Can you work these out from the model? Positions are in its coordinate system, mm. A direction names the side the tool comes from. Give positions to 0.01 mm unless a question says otherwise; leave off trailing zeros. Order: outer loops, then holes, each group sorted by start corner. A loop starts at its lowest first (then second) coordinate and runs counter-clockwise, first axis right, second up. Notation, with made-up numbers: M 58,59.25 L 98,59.25 A23 cw 98,84.25 Z; hole C -3.5,78 d5. An arc over 180 degrees is marked long. Use one line per item in the form item = value. Start each with the question number.
1. I need wall thicknesses on L1, parallel to Y at x = 109, z = 1.3; L2, parallel to X at y = 79.5, z = 2.6; L3, parallel to X at y = 73.5, z = 0.85. Which ranges of each line are inside material? Lowest first, please.
2. Will these pins go through, and if not, where does the flat tip stop? P1, Ø3.5, axis at x = 109, y = 7.96, coming from the -Z side; P2, Ø2, axis at x = 80.5, z = 1, coming from the +Y side.
3. For faces 1 (the face through (73, 53.484, 2)), 2 (the face through (39, -26, 2)), which set-ups out of +Z, -Z, +X, -X, +Y, -Y let a thin tool reach every point of the face, with its end or its side?
4. I want a section at A-A, the plane y = 40. List the corners of the cut face in (x, z) for me.
5. I want a section at C-C, the plane y = 109. List the corners of the cut face in (x, z) for me.
6. We'd pull the mould along Y, two halves only. Please class faces 3 (the face through (106.14, 8.86, 1.97)), 4 (the face through (29, 123.484, 2)), 5 (the face through (141.001, 48, 2)): +Y half, -Y half, draft (parallel to the pull), parting line (faces both ways), or undercut.
7. I want a section at D-D, the plane z = 2. Count the separate pieces of the cut face and the enclosed holes in it, and give its area (3 significant figures).
8. I want a section at B-B, the plane x = 36. List the corners of the cut face in (y, z) for me, and give its area (3 significant figures).
```python
from build123d import *

# Parameters (mm, degrees)
SKETCH_1_R          = 2
EXTRUDE_1_DEPTH     = 4
SKETCH_2_R          = 2
CUT_EXTRUDE_1_DEPTH = 26
EXTRUDE_3_DEPTH     = 4
FILLET_1_R          = 4
FILLET_2_R          = 4
SKETCH_5_W          = 10
SKETCH_5_H          = 14
EXTRUDE_4_DEPTH     = 4
FILLET_3_R          = 4
FILLET_1_2_DEPTH    = 4
CUT_EXTRUDE_2_DEPTH = 10
SKETCH_7_R          = 3
CUT_EXTRUDE_3_DEPTH = 10
CUT_EXTRUDE_4_DEPTH = 10
SKETCH_9_W          = 20
SKETCH_9_H          = 70
SKETCH_9_R          = 3
CUT_EXTRUDE_5_DEPTH = 10
CUT_EXTRUDE_6_DEPTH = 10


with BuildPart() as part:
    # 草图1 → 凸台-拉伸1 (new body)
    with BuildSketch(Plane.XY):
        with BuildLine():
            Line((0, -30), (0, 87))
            Line((0, 87), (-8, 87))
            Line((-8, 87), (-8, 95))
            Line((-8, 95), (0, 95))
            Line((0, 95), (0, 155))
            Line((0, 155), (-20, 155))
            Line((-20, 155), (-20, 180))
            Line((-20, 180), (-8, 180))
            ThreePointArc((-8, 180), (-0.928932188, 182.928932188), (2, 190))
            Line((2, 190), (2, 212))
            Line((2, 212), (10, 212))
            Line((10, 212), (10, 190))
            ThreePointArc((10, 190), (12.928932188, 182.928932188), (20, 180))
            Line((20, 180), (72.5, 180))
            Line((72.5, 180), (125, 180))
            ThreePointArc((125, 180), (132.071067812, 182.928932188), (135, 190))
            Line((135, 190), (135, 212))
            Line((135, 212), (143, 212))
            Line((143, 212), (143, 190))
            ThreePointArc((143, 190), (145.928932188, 182.928932188), (153, 180))
            Line((153, 180), (165, 180))
            Line((165, 180), (165, 155))
            Line((165, 155), (145, 155))
            Line((145, 155), (145, 95))
            Line((145, 95), (153, 95))
            Line((153, 95), (153, 87))
            Line((153, 87), (145, 87))
            Line((145, 87), (145, -30))
            Line((145, -30), (0, -30))
        make_face()
        with Locations((139, 208)):
            Circle(SKETCH_1_R, mode=Mode.SUBTRACT)
        with Locations(Location((149, 91, 0), (0, 0, 180))):
            Circle(SKETCH_1_R, mode=Mode.SUBTRACT)
        with Locations(Location((9, 40, 0), (0, 0, 180))):
            Circle(SKETCH_1_R, mode=Mode.SUBTRACT)
        with Locations(Location((9, 120, 0), (0, 0, 180))):
            Circle(SKETCH_1_R, mode=Mode.SUBTRACT)
        with Locations((-4, 91)):
            Circle(SKETCH_1_R, mode=Mode.SUBTRACT)
        with Locations(Location((6, 208, 0), (0, 0, 180))):
            Circle(SKETCH_1_R, mode=Mode.SUBTRACT)
        with Locations((136, 120)):
            Circle(SKETCH_1_R, mode=Mode.SUBTRACT)
        with Locations((136, 40)):
            Circle(SKETCH_1_R, mode=Mode.SUBTRACT)
    extrude(amount=EXTRUDE_1_DEPTH)

    # 草图2 → 切除-拉伸1 (cut)
    with BuildSketch(Plane(origin=(0, 0, 0), x_dir=(-1, 0, 0), z_dir=(0, 0, -1))):
        with Locations((-90.5, 176)):
            Circle(SKETCH_2_R)
        with Locations((-82.5, 176)):
            Circle(SKETCH_2_R)
        with Locations((-62.5, 176)):
            Circle(SKETCH_2_R)
        with Locations((-54.5, 176)):
            Circle(SKETCH_2_R)
    extrude(amount=-CUT_EXTRUDE_1_DEPTH, mode=Mode.SUBTRACT)

    # 草图4 → 凸台-拉伸3 (add)
    with BuildSketch(Plane(origin=(0, 0, 0), x_dir=(-1, 0, 0), z_dir=(0, 0, -1))):
        with BuildLine():
            Line((-102.5, 194), (-102.5, 204.972470671))
            Line((-102.5, 204.972470671), (-99, 215.944941341))
            Line((-99, 215.944941341), (-95.5, 215.944941341))
            ThreePointArc((-95.5, 215.944941341), (-92.121980777, 211.957020041), (-89.03099134, 207.742721229))
            ThreePointArc((-89.03099134, 207.742721229), (-72.5, 199), (-55.96900866, 207.742721229))
            ThreePointArc((-55.96900866, 207.742721229), (-52.878019223, 211.957020041), (-49.5, 215.944941341))
            Line((-49.5, 215.944941341), (-46, 215.944941341))
            Line((-46, 215.944941341), (-42.5, 204.972470671))
            Line((-42.5, 204.972470671), (-42.5, 194))
            Line((-42.5, 194), (-42.5, 180))
            Line((-42.5, 180), (-49.5, 180))
            Line((-49.5, 180), (-49.5, 194))
            Line((-49.5, 194), (-95.5, 194))
            Line((-95.5, 194), (-95.5, 180))
            Line((-95.5, 180), (-102.5, 180))
            Line((-102.5, 180), (-102.5, 194))
        make_face()
    extrude(amount=-EXTRUDE_3_DEPTH)

    # Fillet 1
    fillet_1_edges = [part.edges().sort_by_distance(p)[0] for p in [
        (102.5, 180, 2),
    ]]
    fillet(fillet_1_edges, radius=FILLET_1_R)

    # 圆角2
    fillet_2_edges = [part.edges().sort_by_distance(p)[0] for p in [
        (42.5, 180, 2),
    ]]
    fillet(fillet_2_edges, radius=FILLET_2_R)

    # 草图5 → 凸台-拉伸4 (add)
    with BuildSketch(Plane(origin=(0, 0, 0), x_dir=(-1, 0, 0), z_dir=(0, 0, -1))):
        with Locations((-71.485667886, 187)):
            Rectangle(SKETCH_5_W, SKETCH_5_H)
    extrude(amount=-EXTRUDE_4_DEPTH)

    # 圆角3
    fillet_3_edges = [part.edges().sort_by_distance(p)[0] for p in [
        (0, 95, 2),
    ]]
    fillet(fillet_3_edges, radius=FILLET_3_R)

    # Fillet 1 2: read off the stored shape, not the designer's step
    # Fillet 1 2 outline → Fillet 1 2 (add)
    with BuildSketch(Plane.XY):
        with BuildLine():
            add(Edge.make_bspline(
                [(0, 85), (0, 87), (-2, 87)],
                knots=[0, 0, 0, 1, 1, 1], degree=2, weights=[1, 0.707106781, 1]))
            Line((0, 85), (0, 87))
            Line((0, 87), (-2, 87))
        make_face()
        with BuildLine():
            add(Edge.make_bspline(
                [(145, 97), (145, 95), (147, 95)],
                knots=[0, 0, 0, 1, 1, 1], degree=2, weights=[1, 0.707106781, 1]))
            Line((145, 97), (145, 95))
            Line((145, 95), (147, 95))
        make_face()
        with BuildLine():
            add(Edge.make_bspline(
                [(147, 87), (145, 87), (145, 85)],
                knots=[0, 0, 0, 1, 1, 1], degree=2, weights=[1, 0.707106781, 1]))
            Line((147, 87), (145, 87))
            Line((145, 87), (145, 85))
        make_face()
    extrude(amount=FILLET_1_2_DEPTH)

    # 草图6 → 切除-拉伸2 (cut)
    with BuildSketch(Plane(origin=(0, 0, 0), x_dir=(-1, 0, 0), z_dir=(0, 0, -1))):
        with BuildLine():
            Line((-145, 126), (0, 127))
            ThreePointArc((0, 127), (86.5779564, 788.380122484), (-240.522742442, 207.067348009))
            Line((-240.522742442, 207.067348009), (-145, 126))
        make_face()
        Polygon((-145, 97), (-145, 85), (-184.843069779, 78.009614434), (-187.688323439, 115.332647741), align=None)
        Polygon((0, 85), (0, 99), (22.414932697, 115.332647741), (70.043948421, 78.009614434), align=None)
    extrude(amount=-CUT_EXTRUDE_2_DEPTH, mode=Mode.SUBTRACT)

    # 草图7 → 切除-拉伸3 (cut)
    with BuildSketch(Plane(origin=(0, 0, 0), x_dir=(-1, 0, 0), z_dir=(0, 0, -1))):
        with Locations((-109, 7.960589548)):
            Circle(SKETCH_7_R)
        with Locations((-36, 7.960589548)):
            Circle(SKETCH_7_R)
        with Locations((-109, -26.039410452)):
            Circle(SKETCH_7_R)
        with Locations((-36, -26.039410452)):
            Circle(SKETCH_7_R)
        with Locations((-124.840103492, 79.073280951)):
            Circle(SKETCH_7_R)
        with Locations((-124.840103492, 21.073280951)):
            Circle(SKETCH_7_R)
        with Locations((-95.840103492, 21.073280951)):
            Circle(SKETCH_7_R)
        with Locations((-95.840103492, 79.073280951)):
            Circle(SKETCH_7_R)
        with Locations((-65.68273437, 95.743302343)):
            Circle(SKETCH_7_R)
        with Locations((-65.68273437, 12.743302343)):
            Circle(SKETCH_7_R)
        with Locations((-17.742400545, 17.739740347)):
            Circle(SKETCH_7_R)
        with Locations((-17.742400545, 92.739740347)):
            Circle(SKETCH_7_R)
    extrude(amount=-CUT_EXTRUDE_3_DEPTH, mode=Mode.SUBTRACT)

    # 草图8 → 切除-拉伸4 (cut)
    with BuildSketch(Plane(origin=(0, 0, 0), x_dir=(-1, 0, 0), z_dir=(0, 0, -1))):
        Polygon((-154.568758674, 123.48356313), (9.260166048, 123.48356313), (22.383573851, 133.739706362), (-120.787265427, 138.710916059), align=None)
    extrude(amount=-CUT_EXTRUDE_4_DEPTH, mode=Mode.SUBTRACT)

    # 草图9 → 切除-拉伸5 (cut)
    # profile 1 of 2: a face of its own
    with BuildSketch(Plane(origin=(0, 0, 0), x_dir=(-1, 0, 0), z_dir=(0, 0, -1))):
        with Locations((-82.5, 88.48356313)):
            Rectangle(SKETCH_9_W, SKETCH_9_H)
    # profile 2 of 2: a face of its own
    with BuildSketch(Plane(origin=(0, 0, 0), x_dir=(-1, 0, 0), z_dir=(0, 0, -1))):
        with Locations((-62.5, 88.48356313)):
            Rectangle(SKETCH_9_W, SKETCH_9_H)
        with Locations((-65.68273437, 95.743302343)):
            Circle(SKETCH_9_R, mode=Mode.SUBTRACT)
    extrude(amount=-CUT_EXTRUDE_5_DEPTH, mode=Mode.SUBTRACT)

    # 草图10 → 切除-拉伸6 (cut)
    with BuildSketch(Plane(origin=(0, 0, 0), x_dir=(-1, 0, 0), z_dir=(0, 0, -1))):
        Polygon((-141.001388933, 153.448037881), (-141.001388933, -56.355097375), (-194.104207941, 53.872664694), align=None)
        Polygon((-4, 153.448037881), (-4, -50.760982065), (2.911690677, -47.431237796), (83.451298672, 119.6813615), align=None)
    extrude(amount=-CUT_EXTRUDE_6_DEPTH, mode=Mode.SUBTRACT)


solid = part.part
```
Check result:
q1.L1 = -30 to -29.04, -23.04 to 4.96, 10.96 to 123.48
q1.L2 = 4 to 52.5, 92.5 to 92.87, 98.81 to 121.87, 127.81 to 141
q1.L3 = 4 to 52.5, 92.5 to 141
q2.P1 = through
q2.P2 = 53.48
q3.face_1 = +Z, -Z, +Y
q3.face_2 = +Z, -Z
q4.outline = M 4,0 L 7,0 L 7,4 L 4,4 Z; M 11,0 L 134,0 L 134,4 L 11,4 Z; M 138,0 L 141,0 L 141,4 L 138,4 Z
q5.outline = M 4,0 L 52.5,0 L 52.5,4 L 4,4 Z; M 92.5,0 L 141,0 L 141,4 L 92.5,4 Z
q6.face_3 = undercut
q6.face_4 = +Y half
q6.face_5 = draft
q7.separate_pieces = 1
q7.enclosed_holes = 15
q7.area = 17,900 mm2
q8.outline = M -30,0 L -29.04,0 L -29.04,4 L -30,4 Z; M -23.04,0 L 4.96,0 L 4.96,4 L -23.04,4 Z; M 10.96,0 L 123.48,0 L 123.48,4 L 10.96,4 Z
q8.area = 566 mm2
